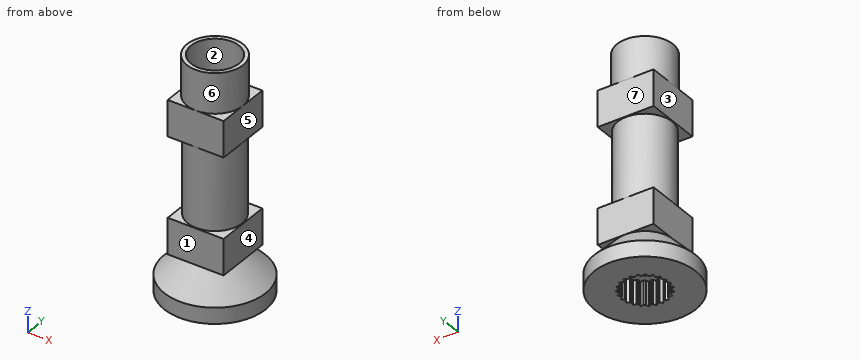
```python
from build123d import *

# Parameters (mm, degrees)
SKETCH_2_R               = 3.5
EXTRUDE_3_DEPTH          = 19
SKETCH_1_R               = 6.35
EXTRUDE_4_DEPTH          = 2
SKETCH_5_R               = 3.5
EXTRUDE_5_DEPTH          = 2
SKETCH_6_R               = 2.75
CUT_EXTRUDE_1_DEPTH      = 3
SKETCH_7_R               = 1.8
CUT_EXTRUDE_2_DEPTH      = 28.507180927
SKETCH_8_R               = 3
CUT_EXTRUDE_3_DEPTH      = 23
CUT_EXTRUDE_5_DEPTH      = 3
SKETCH_14_W              = 7
SKETCH_14_H              = 7
SKETCH_14_R              = 3.4
EXTRUDE_7_DEPTH          = 19
SKETCH_16_W              = 7
SKETCH_16_H              = 7
SKETCH_16_R              = 3.4
CUT_EXTRUDE_6_DEPTH      = 5
CUT_EXTRUDE_6_DEPTH_BACK = 5
SKETCH_17_R              = 3
SKETCH_17_R_2            = 1.8
EXTRUDE_8_DEPTH          = 14


with BuildPart() as part:
    # ｽｹｯﾁ2 → ﾎﾞｽ - 押し出し3 (new body)
    with BuildSketch(Plane.XY.offset(5)):
        with Locations(Location((0, 0, 0), (0, 0, 180))):
            Circle(SKETCH_2_R)
    extrude(amount=EXTRUDE_3_DEPTH)


with BuildPart() as body_2:
    # ｽｹｯﾁ1 → ﾎﾞｽ - 押し出し4 (new body)
    with BuildSketch(Plane.XY):
        Circle(SKETCH_1_R)
    extrude(amount=EXTRUDE_4_DEPTH)


    add(part.part)  # loft_1 joins it to this body
    # loft from a face of the part (loft_1)
    loft([body_2.faces().sort_by_distance((0, 0, 2))[0], body_2.faces().sort_by_distance((0, 0, 5))[0]])



with BuildPart() as body_3:
    # ｽｹｯﾁ5 → ﾎﾞｽ - 押し出し5 (new body)
    with BuildSketch(Plane.XY.offset(29)):
        Circle(SKETCH_5_R)
    extrude(amount=-EXTRUDE_5_DEPTH)


with BuildPart() as body_2_1:
    add(body_2.part)

    add(body_3.part)  # loft_2 joins it to this body
    # loft from a face of the part (loft_2)
    loft([body_2_1.faces().sort_by_distance((0, 0, 24))[0], body_2_1.faces().sort_by_distance((0, 0, 27))[0]])

    # ｽｹｯﾁ6 → ｶｯﾄ - 押し出し1 (cut)
    with BuildSketch(Plane(origin=(0, 0, 0), x_dir=(-1, 0, 0), z_dir=(0, 0, -1))):
        Circle(SKETCH_6_R)
    extrude(amount=-CUT_EXTRUDE_1_DEPTH, mode=Mode.SUBTRACT)

    # ｽｹｯﾁ7 → ｶｯﾄ - 押し出し2 (cut, through all)
    with BuildSketch(Plane(origin=(0, 0, 3), x_dir=(-1, 0, 0), z_dir=(0, 0, -1))):
        Circle(SKETCH_7_R)
    extrude(amount=-CUT_EXTRUDE_2_DEPTH, mode=Mode.SUBTRACT)

    # ｽｹｯﾁ8 → ｶｯﾄ - 押し出し3 (cut)
    with BuildSketch(Plane.XY.offset(29)):
        Circle(SKETCH_8_R)
    extrude(amount=-CUT_EXTRUDE_3_DEPTH, mode=Mode.SUBTRACT)

    # ｽｹｯﾁ12 → ｶｯﾄ - 押し出し5 (cut)
    with BuildSketch(Plane(origin=(0, 0, 0), x_dir=(-1, 0, 0), z_dir=(0, 0, -1))):
        with BuildLine():
            Line((0.208139361, 3.042889746), (-0.062598794, 2.749287433))
            ThreePointArc((-0.062598794, 2.749287433), (0.187666637, 2.743589115), (0.436377003, 2.715156554))
            Line((0.436377003, 2.715156554), (0.208139361, 3.042889746))
        make_face()
        with BuildLine():
            Line((1.021382817, 2.873895812), (0.681471411, 2.66422535))
            ThreePointArc((0.681471411, 2.66422535), (0.920918933, 2.591217536), (1.152735431, 2.496738077))
            Line((1.152735431, 2.496738077), (1.021382817, 2.873895812))
        make_face()
        with BuildLine():
            Line((1.758874982, 2.491758174), (1.375, 2.38156986))
            ThreePointArc((1.375, 2.38156986), (1.585870886, 2.246667206), (1.783600746, 2.093147959))
            Line((1.783600746, 2.093147959), (1.758874982, 2.491758174))
        make_face()
        with BuildLine():
            Line((2.365919437, 1.92481823), (1.966551129, 1.922284229))
            ThreePointArc((1.966551129, 1.922284229), (2.133206049, 1.735491847), (2.282184553, 1.534318633))
            Line((2.282184553, 1.534318633), (2.365919437, 1.92481823))
        make_face()
        with BuildLine():
            Line((2.79749447, 1.215123324), (2.412252157, 1.320431571))
            ThreePointArc((2.412252157, 1.320431571), (2.522331079, 1.095602997), (2.611509172, 0.861695912))
            Line((2.611509172, 0.861695912), (2.79749447, 1.215123324))
        make_face()
        with BuildLine():
            Line((3.021592135, 0.41530828), (2.679047477, 0.620648543))
            ThreePointArc((2.679047477, 0.620648543), (2.724386352, 0.374458285), (2.747150103, 0.125165148))
            Line((2.747150103, 0.125165148), (3.021592135, 0.41530828))
        make_face()
        with BuildLine():
            Line((3.021592135, -0.41530828), (2.747150103, -0.125165148))
            ThreePointArc((2.747150103, -0.125165148), (2.724386352, -0.374458285), (2.679047477, -0.620648543))
            Line((2.679047477, -0.620648543), (3.021592135, -0.41530828))
        make_face()
        with BuildLine():
            Line((2.79749447, -1.215123324), (2.611509172, -0.861695912))
            ThreePointArc((2.611509172, -0.861695912), (2.522331079, -1.095602997), (2.412252157, -1.320431571))
            Line((2.412252157, -1.320431571), (2.79749447, -1.215123324))
        make_face()
        with BuildLine():
            Line((2.365919437, -1.92481823), (2.282184553, -1.534318633))
            ThreePointArc((2.282184553, -1.534318633), (2.133206049, -1.735491847), (1.966551129, -1.922284229))
            Line((1.966551129, -1.922284229), (2.365919437, -1.92481823))
        make_face()
        with BuildLine():
            Line((1.758874982, -2.491758174), (1.783600746, -2.093147959))
            ThreePointArc((1.783600746, -2.093147959), (1.585870886, -2.246667206), (1.375, -2.38156986))
            Line((1.375, -2.38156986), (1.758874982, -2.491758174))
        make_face()
        with BuildLine():
            Line((1.021382817, -2.873895812), (1.152735431, -2.496738077))
            ThreePointArc((1.152735431, -2.496738077), (0.920918933, -2.591217536), (0.681471411, -2.66422535))
            Line((0.681471411, -2.66422535), (1.021382817, -2.873895812))
        make_face()
        with BuildLine():
            Line((0.208139361, -3.042889746), (0.436377003, -2.715156554))
            ThreePointArc((0.436377003, -2.715156554), (0.187666637, -2.743589115), (-0.062598794, -2.749287433))
            Line((-0.062598794, -2.749287433), (0.208139361, -3.042889746))
        make_face()
        with BuildLine():
            Line((-0.62054084, -2.986206467), (-0.312345512, -2.73220429))
            ThreePointArc((-0.312345512, -2.73220429), (-0.559504036, -2.692481241), (-0.802026334, -2.630447445))
            Line((-0.802026334, -2.630447445), (-0.62054084, -2.986206467))
        make_face()
        with BuildLine():
            Line((-1.403198365, -2.708049916), (-1.037902788, -2.546616933))
            ThreePointArc((-1.037902788, -2.546616933), (-1.265178854, -2.441684351), (-1.481971249, -2.316519203))
            Line((-1.481971249, -2.316519203), (-1.403198365, -2.708049916))
        make_face()
        with BuildLine():
            Line((-2.081787087, -2.229049691), (-1.686483563, -2.172158648))
            ThreePointArc((-1.686483563, -2.172158648), (-1.877021144, -2.009798902), (-2.052005136, -1.830785329))
            Line((-2.052005136, -1.830785329), (-2.081787087, -2.229049691))
        make_face()
        with BuildLine():
            Line((-2.605979184, -1.584731048), (-2.209985568, -1.636601293))
            ThreePointArc((-2.209985568, -1.636601293), (-2.349653363, -1.428855863), (-2.46985119, -1.209270483))
            Line((-2.46985119, -1.209270483), (-2.605979184, -1.584731048))
        make_face()
        with BuildLine():
            Line((-2.936897726, -0.822880152), (-2.569583052, -0.979664707))
            ThreePointArc((-2.569583052, -0.979664707), (-2.64802254, -0.741941121), (-2.704519679, -0.498069577))
            Line((-2.704519679, -0.498069577), (-2.936897726, -0.822880152))
        make_face()
        with BuildLine():
            Line((-3.05, 0), (-2.738606317, -0.250070871))
            ThreePointArc((-2.738606317, -0.250070871), (-2.75, 0), (-2.738606317, 0.250070871))
            Line((-2.738606317, 0.250070871), (-3.05, 0))
        make_face()
        with BuildLine():
            Line((-2.936897726, 0.822880152), (-2.704519679, 0.498069577))
            ThreePointArc((-2.704519679, 0.498069577), (-2.64802254, 0.741941121), (-2.569583052, 0.979664707))
            Line((-2.569583052, 0.979664707), (-2.936897726, 0.822880152))
        make_face()
        with BuildLine():
            Line((-2.605979184, 1.584731048), (-2.46985119, 1.209270483))
            ThreePointArc((-2.46985119, 1.209270483), (-2.349653363, 1.428855863), (-2.209985568, 1.636601293))
            Line((-2.209985568, 1.636601293), (-2.605979184, 1.584731048))
        make_face()
        with BuildLine():
            Line((-2.081787087, 2.229049691), (-2.052005136, 1.830785329))
            ThreePointArc((-2.052005136, 1.830785329), (-1.877021144, 2.009798902), (-1.686483563, 2.172158648))
            Line((-1.686483563, 2.172158648), (-2.081787087, 2.229049691))
        make_face()
        with BuildLine():
            Line((-1.403198365, 2.708049916), (-1.481971249, 2.316519203))
            ThreePointArc((-1.481971249, 2.316519203), (-1.265178854, 2.441684351), (-1.037902788, 2.546616933))
            Line((-1.037902788, 2.546616933), (-1.403198365, 2.708049916))
        make_face()
        with BuildLine():
            Line((-0.62054084, 2.986206467), (-0.802026334, 2.630447445))
            ThreePointArc((-0.802026334, 2.630447445), (-0.559504036, 2.692481241), (-0.312345512, 2.73220429))
            Line((-0.312345512, 2.73220429), (-0.62054084, 2.986206467))
        make_face()
    extrude(amount=-CUT_EXTRUDE_5_DEPTH, mode=Mode.SUBTRACT)

    # ｽｹｯﾁ14 → ﾎﾞｽ - 押し出し7 (add)
    with BuildSketch(Plane.XY.offset(24)):
        Rectangle(SKETCH_14_W, SKETCH_14_H)
        Circle(SKETCH_14_R, mode=Mode.SUBTRACT)
    extrude(amount=-EXTRUDE_7_DEPTH)

    # ｽｹｯﾁ16 → ｶｯﾄ - 押し出し6 (cut, two sides)
    with BuildSketch(Plane.XY.offset(14.5)) as cut_extrude_6_sk:
        Rectangle(SKETCH_16_W, SKETCH_16_H)
        Circle(SKETCH_16_R, mode=Mode.SUBTRACT)
    extrude(amount=CUT_EXTRUDE_6_DEPTH, mode=Mode.SUBTRACT)
    extrude(cut_extrude_6_sk.sketch, amount=-CUT_EXTRUDE_6_DEPTH_BACK, mode=Mode.SUBTRACT)

    # ｽｹｯﾁ17 → ﾎﾞｽ - 押し出し8 (add)
    with BuildSketch(Plane.XY.offset(6)):
        Circle(SKETCH_17_R)
        with Locations(Location((0, 0, 0), (0, 0, 180))):
            Circle(SKETCH_17_R_2, mode=Mode.SUBTRACT)
    extrude(amount=EXTRUDE_8_DEPTH)


solid = body_2_1.part
```
The model under review builds one solid part; all positions refer to its coordinate system, in mm. Face numbers are marked on the shaded views. A direction names the side the tool comes from. Coordinates: 2 decimals unless noted, no trailing zeros. Write each loop counter-clockwise with the first axis right and the second up, starting at its lowest first coordinate (ties: lowest second). Pieces come first, ordered by that corner, then holes. Notation, with made-up numbers: (26.25, -26) - (64.25, -26) arc R26 cw to (64.25, -10) - close; hole circle Ø1 at (89, -22). An arc over 180 degrees is marked (long way). Answer in a Markdown table with one row per item. Add a question column.
Q1. To check wall thickness, follow line 1 along Y through (x, z) = (0, 23); line 2 along Y through (x, z) = (0, 16); line 3 along X through (y, z) = (0, 7). State the ranges of each line that lie inside material, in increasing order. Write a range as from..to.
Q2. For the marked faces 5, 6 and 7, list the 3-axis set-ups (+Z, -Z, +X, -X, +Y, -Y) from which the entire face can be reached by the end or side of a thin tool; tool diameter is ignored.
Q3. Clearance check with flat-ended pins moving along their axes: pin 1 (3.5 mm diameter, centred on y = -1.5, z = 21, fed in from +X); pin 2 (2 mm diameter, centred on y = 0, z = 7.5, fed in from -X); pin 3 (2 mm diameter, centred on x = -0.5, z = 22, fed in from -Y). State where each tip first meets the part, or that it passes through.
Q4. Consider section A-A on z = 8.5. Give the boundary of the cut face in (x, y), then the cut area to 3 significant figures.
Q5. Draft analysis for pull direction X (two halves, no side actions). For the marked faces 1, 2, 3 and 4, state which applies: +X half, -X half, draft (parallel to the pull), parting line (faces both ways), or undercut.
Q6. Consider section B-B on z = 22. Give the boundary of the cut face in (x, y), then the cut area to 3 significant figures.
Answers below:
| question | item | result |
|---|---|---|
| 1 | line 1 | -3.5..-3, 3..3.5 |
| 1 | line 2 | -3.4..-1.8, 1.8..3.4 |
| 1 | line 3 | -3.5..-1.8, 1.8..3.5 |
| 2 | face 5 | +Z, +X, +Y, -Y |
| 2 | face 6 | +Z |
| 2 | face 7 | +Z, +X, -X, +Y |
| 3 | pin 1 | x = 3.5 |
| 3 | pin 2 | x = -3.5 |
| 3 | pin 3 | y = -3.5 |
| 4 | outline | (-3.5, -3.5) - (3.5, -3.5) - (3.5, 3.5) - (-3.5, 3.5) - close; hole circle Ø3.6 at (0, 0) |
| 4 | area | 38.8 mm² |
| 5 | face 1 | draft |
| 5 | face 2 | undercut |
| 5 | face 3 | -X half |
| 5 | face 4 | +X half |
| 6 | outline | (-3.5, -3.5) - (3.5, -3.5) - (3.5, 3.5) - (-3.5, 3.5) - close; hole circle Ø6 at (0, 0) |
| 6 | area | 20.7 mm² |
